Check sheet for the modelled part. Datum: model origin and axes. Units: mm. Face numbers are marked on the shaded views. A direction names the side the tool comes from. Coordinates: 2 decimals unless noted, no trailing zeros. Order: outer loops, then holes, each group sorted by start corner. A loop starts at its lowest first (then second) coordinate and runs counter-clockwise, first axis right, second up.
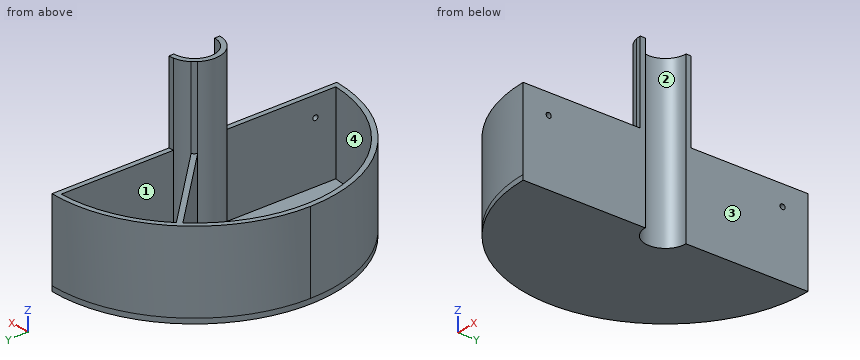
from build123d import *

# Parameters (mm, degrees)
F1_DEPTH = 3.175
F3_DEPTH = 50.8
F5_DEPTH = 50.8
F6_R     = 1.5875
F7_DEPTH = 3.175


with BuildPart() as f1:
    # F0 (on Top) → F1 (new body)
    with BuildSketch(Plane.XY):
        with BuildLine():
            Line((0, 12.7), (0, 88.9))
            ThreePointArc((0, 88.9), (-88.9, 0), (0, -88.9))
            Line((0, -88.9), (0, -12.7))
            ThreePointArc((0, -12.7), (-12.7, 0), (0, 12.7))
        make_face()
    extrude(amount=F1_DEPTH)

    # F2 (on face) → F3 (join)
    with BuildSketch(Plane.XY.offset(3.175)):
        with BuildLine():
            ThreePointArc((0, -12.7), (-12.7, 0), (0, 12.7))
            Line((0, 12.7), (0, 88.9))
            ThreePointArc((0, 88.9), (-62.861793, 62.861793), (-88.9, 0))
            ThreePointArc((-88.9, 0), (-62.861793, -62.861793), (0, -88.9))
            Line((0, -88.9), (0, -12.7))
        make_face()
        with BuildLine():
            ThreePointArc((-13.243587, 8.753459), (-14.666588, -6.075099), (-3.175, -15.55426))
            Line((-3.175, -15.55426), (-3.175, -85.666184))
            ThreePointArc((-3.175, -85.666184), (-79.199573, -32.805537), (-62.820203, 58.330075))
            Line((-62.820203, 58.330075), (-13.243587, 8.753459))
        make_face(mode=Mode.SUBTRACT)
        with BuildLine():
            Line((-3.175, 85.666184), (-3.175, 15.55426))
            ThreePointArc((-3.175, 15.55426), (-7.51846, 13.981716), (-11.22532, 11.22532))
            Line((-11.22532, 11.22532), (-60.616729, 60.616729))
            ThreePointArc((-60.616729, 60.616729), (-34.26682, 78.578373), (-3.175, 85.666184))
        make_face(mode=Mode.SUBTRACT)
    extrude(amount=F3_DEPTH)

    # F4 (on face) → F5 (join)
    with BuildSketch(Plane.XY.offset(53.975)):
        with BuildLine():
            ThreePointArc((0, -12.7), (-12.7, 0), (0, 12.7))
            Line((0, 12.7), (0, 15.875))
            ThreePointArc((0, 15.875), (-1.59558, 15.794611), (-3.175, 15.55426))
            ThreePointArc((-3.175, 15.55426), (-7.51846, 13.981716), (-11.22532, 11.22532))
            ThreePointArc((-11.22532, 11.22532), (-12.296722, 10.040232), (-13.243587, 8.753459))
            ThreePointArc((-13.243587, 8.753459), (-14.666588, -6.075099), (-3.175, -15.55426))
            ThreePointArc((-3.175, -15.55426), (-1.59558, -15.794611), (0, -15.875))
            Line((0, -15.875), (0, -12.7))
        make_face()
    extrude(amount=F5_DEPTH)

    # F6 (on face) → F7 (cut)
    with BuildSketch(Plane(origin=(-3.175, 0, 0), x_dir=(0, -1, 0), z_dir=(-1, 0, 0))):
        with Locations((72.966184, 41.275)):
            Circle(F6_R)
        with Locations((-72.966184, 41.275)):
            Circle(F6_R)
    extrude(amount=-F7_DEPTH, mode=Mode.SUBTRACT)


solid = f1.part
(1) Cross-section at C-C (x = -18.5). Enter the section's corners in (y, z) (3 decimals), and give its area (3 significant figures).
Filled in:
outline: (-86.954, 0) - (86.954, 0) - (86.954, 53.975) - (83.705, 53.975) - (83.705, 3.175) - (18.5, 3.175) - (18.5, 53.975) - (14.01, 53.975) - (14.01, 3.175) - (-83.705, 3.175) - (-83.705, 53.975) - (-86.954, 53.975) - close
area: 1,110 mm2
(2) Cross-section at B-B (z = 69). Enter the section's corners in (x, y) (3 decimals), and give its area (3 significant figures).
Filled in:
outline: (-13.244, 8.753) arc R15.875 ccw to (-3.175, -15.554) arc R15.875 ccw to (0, -15.875) - (0, -12.7) arc R12.7 cw to (0, 12.7) - (0, 15.875) arc R15.875 ccw to (-3.175, 15.554) arc R15.875 ccw to (-11.225, 11.225) arc R15.875 ccw to start
area: 143 mm2
(3) Thickness scan on probe 1 along X at (y, z) = (47, 46) (3 decimals); probe 2 along X at (y, z) = (46.5, 26) (3 decimals); probe 3 along Y at (x, z) = (-17.5, 28). Record the ranges inside material, lowest first.
Filled in:
probe 1: x = -75.46 to -71.692, -51.49 to -47, -3.175 to 0
probe 2: x = -75.769 to -72.018, -50.99 to -46.5, -3.175 to 0
probe 3: y = -87.16 to -83.92, 13.01 to 17.5, 83.92 to 87.16
(4) Tool access check on the marked faces 1 and 2. Record the directions out of +Z, -Z, +X, -X, +Y, -Y that give a thin tool (end or side, any length) a straight path to the whole face; none if there is none.
Filled in:
face 1: +Z
face 2: +Z, -Z, +X
(5) Cross-section at D-D (y = 53.5). Enter the section's corners in (x, z) (3 decimals).
Filled in:
outline: (-71, 0) - (0, 0) - (0, 53.975) - (-3.175, 53.975) - (-3.175, 3.175) - (-53.5, 3.175) - (-53.5, 53.975) - (-57.99, 53.975) - (-57.99, 3.175) - (-66.982, 3.175) - (-66.982, 53.975) - (-71, 53.975) - close
(6) Go/stop test with flat-tipped pins: P1, Ø1, axis at x = -13.5, z = 75, coming from the +Y side; P2, Ø3, axis at x = -13, y = -56.5, coming from the +Z side (3 decimals); P3, Ø6, axis at x = -25, y = 17, coming from the +Z side (3 decimals). Record where each tip stops, or that it passes through.
Filled in:
P1: stops at y = 9.11
P2: stops at z = 3.175
P3: stops at z = 53.975
(7) Release check for a two-part mould opening along Y. For the marked faces 3 and 4 record: +Y half, -Y half, draft (parallel to the pull), parting line (faces both ways), or undercut.
Filled in:
face 3: draft
face 4: undercut
(8) Cross-section at A-A (z = 9.5). Enter the section's corners in (x, y) (3 decimals), and give its area (3 significant figures).
Filled in:
outline: (-88.9, 0) arc R88.9 ccw to (0, -88.9) - (0, -12.7) arc R12.7 cw to (0, 12.7) - (0, 88.9) arc R88.9 ccw to start; hole (-62.82, 58.33) arc R85.725 ccw to (-3.175, -85.666) - (-3.175, -15.554) arc R15.875 cw to (-13.244, 8.753) - close; hole (-60.617, 60.617) - (-11.225, 11.225) arc R15.875 cw to (-3.175, 15.554) - (-3.175, 85.666) arc R85.725 ccw to start
area: 1,680 mm2
